Check sheet for the modelled part. Datum: model origin and axes. Units: mm. Face numbers are marked on the shaded views. A direction names the side the tool comes from. Give positions to 0.01 mm unless a question says otherwise; leave off trailing zeros. Write each loop counter-clockwise with the first axis right and the second up, starting at its lowest first coordinate (ties: lowest second). Pieces come first, ordered by that corner, then holes. Notation, with made-up numbers: (-6, 2.25) -> (37, 2.25) arc R17 ccw to (37, 17.25) -> close; hole circle Ø10 at (39.5, 88). An arc over 180 degrees is marked (long way). Return JSON: item names as keys, results as strings.
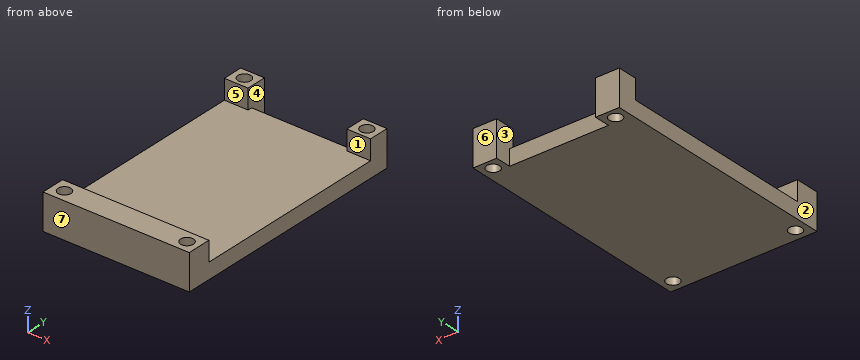
from build123d import *

# Parameters (mm, degrees)
SKETCH1_R           = 3.25
BOSS_EXTRUDE1_DEPTH = 8
SKETCH4_R           = 3.25
BOSS_EXTRUDE3_DEPTH = 10
BOSS_EXTRUDE4_DEPTH = 54
BOSS_EXTRUDE5_DEPTH = 2
BOSS_EXTRUDE6_DEPTH = 2
BOSS_EXTRUDE7_DEPTH = 2
BOSS_EXTRUDE8_DEPTH = 2
SKETCH10_W          = 74
SKETCH10_H          = 18
BOSS_EXTRUDE9_DEPTH = 2


with BuildPart() as part:
    # Sketch1 → Boss-Extrude1 (new body)
    with BuildSketch(Plane.XY):
        Polygon((-27, 52.55), (-27, 60.55), (-35, 60.55), (-35, -60.55), (-27, -60.55), (-27, -52.55), (27, -52.55), (27, -60.55), (35, -60.55), (35, 60.55), (27, 60.55), (27, 52.55), align=None)
        with Locations((31, 55.45)):
            Circle(SKETCH1_R, mode=Mode.SUBTRACT)
        with Locations((-31, 55.45)):
            Circle(SKETCH1_R, mode=Mode.SUBTRACT)
        with Locations((-31, -56.55)):
            Circle(SKETCH1_R, mode=Mode.SUBTRACT)
        with Locations((31, -56.55)):
            Circle(SKETCH1_R, mode=Mode.SUBTRACT)
    extrude(amount=BOSS_EXTRUDE1_DEPTH)

    # Sketch4 → Boss-Extrude3 (add)
    # profile 1 of 4: a face of its own
    with BuildSketch(Plane.XY.offset(8)):
        Polygon((-27, 60.55), (-35, 60.55), (-35, 50.35), (-27, 50.35), (-27, 52.55), align=None)
        with Locations((-31, 55.45)):
            Circle(SKETCH4_R, mode=Mode.SUBTRACT)
    # profile 2 of 4: a face of its own
    with BuildSketch(Plane.XY.offset(8)):
        Polygon((35, 50.35), (35, 60.55), (27, 60.55), (27, 52.55), (27, 50.35), align=None)
        with Locations((31, 55.45)):
            Circle(SKETCH4_R, mode=Mode.SUBTRACT)
    # profile 3 of 4: a face of its own
    with BuildSketch(Plane.XY.offset(8)):
        Polygon((35, -60.55), (35, -50.35), (27, -50.35), (27, -52.55), (27, -60.55), align=None)
        with Locations((31, -56.55)):
            Circle(SKETCH4_R, mode=Mode.SUBTRACT)
    # profile 4 of 4: a face of its own
    with BuildSketch(Plane.XY.offset(8)):
        Polygon((-27, -50.35), (-35, -50.35), (-35, -60.55), (-27, -60.55), (-27, -52.55), align=None)
        with Locations((-31, -56.55)):
            Circle(SKETCH4_R, mode=Mode.SUBTRACT)
    extrude(amount=BOSS_EXTRUDE3_DEPTH)

    # Sketch5 → Boss-Extrude4 (add)
    with BuildSketch(Plane(origin=(-27, 0, 0), x_dir=(0, 0, -1), z_dir=(1, 0, 0))):
        Polygon((-18, -50.35), (-8, -50.35), (-8, -52.55), (0, -52.55), (0, -60.55), (-18, -60.55), align=None)
    extrude(amount=BOSS_EXTRUDE4_DEPTH)

    # Sketch6 → Boss-Extrude5 (add)
    with BuildSketch(Plane(origin=(35, 0, 0), x_dir=(0, 0, -1), z_dir=(1, 0, 0))):
        Polygon((0, -60.55), (0, 60.55), (-18, 60.55), (-18, 50.35), (-8, 50.35), (-8, -50.35), (-18, -50.35), (-18, -60.55), align=None)
    extrude(amount=BOSS_EXTRUDE5_DEPTH)

    # Sketch7 → Boss-Extrude6 (add)
    with BuildSketch(Plane.ZY.offset(-27)):
        Polygon((0, 60.55), (0, 52.55), (8, 52.55), (8, 50.35), (18, 50.35), (18, 60.55), align=None)
    extrude(amount=BOSS_EXTRUDE6_DEPTH)

    # Sketch8 → Boss-Extrude7 (add)
    with BuildSketch(Plane.ZY.offset(35)):
        Polygon((0, 60.55), (0, -60.55), (18, -60.55), (18, -50.35), (8, -50.35), (8, 50.35), (18, 50.35), (18, 60.55), align=None)
    extrude(amount=BOSS_EXTRUDE7_DEPTH)

    # Sketch9 → Boss-Extrude8 (add)
    with BuildSketch(Plane(origin=(-27, 0, 0), x_dir=(0, 0, -1), z_dir=(1, 0, 0))):
        Polygon((0, 52.55), (0, 60.55), (-18, 60.55), (-18, 50.35), (-8, 50.35), (-8, 52.55), align=None)
    extrude(amount=BOSS_EXTRUDE8_DEPTH)

    # Sketch10 → Boss-Extrude9 (add)
    with BuildSketch(Plane.XZ.offset(60.55)):
        with Locations((0, 9)):
            Rectangle(SKETCH10_W, SKETCH10_H)
    extrude(amount=BOSS_EXTRUDE9_DEPTH)


solid = part.part
(1) Set-up check for the marked faces 1, 2 and 3: record each of +Z, -Z, +X, -X, +Y, -Y from which the full face is reachable in a straight line by a thin tool's end or side.
Reply:
{"face 1": "+Z, +X, -X", "face 2": "+Z, -Z, -X, +Y, -Y", "face 3": "+Z, +Y"}
(2) Depth check by flat-ended pin: pin 1 Ø6 at (x, y) = (31, 55.45) entering from -Z; pin 2 Ø8 at (x, z) = (-5, 11.5) entering from +Y; pin 3 Ø4 at (x, y) = (19.5, -15) entering from +Z. Enter the tip coordinate at first touch or a pass-through.
Reply:
{"pin 1": "through", "pin 2": "y = 52.55", "pin 3": "z = 8"}
(3) Cross-section at A-A on x = 31. Enter the section's corners in (y, z), then the cut area to 3 significant figures.
Reply:
{"outline": "(-62.55, 0) -> (-59.8, 0) -> (-59.8, 18) -> (-62.55, 18) -> close; (-53.3, 0) -> (52.2, 0) -> (52.2, 18) -> (50.35, 18) -> (50.35, 8) -> (-50.35, 8) -> (-50.35, 18) -> (-53.3, 18) -> close; (58.7, 0) -> (60.55, 0) -> (60.55, 18) -> (58.7, 18) -> close", "area": "975 mm^2"}
(4) Thickness scan on L1, parallel to Y at x = -31, z = 5.75; L2, parallel to Y at x = -31, z = 8.5; L3, parallel to Y at x = 30, z = 9. Record the ranges inside material, lowest first.
Reply:
{"L1": "-62.55 to -59.8, -53.3 to 52.2, 58.7 to 60.55", "L2": "-62.55 to -59.8, -53.3 to -50.35, 50.35 to 52.2, 58.7 to 60.55", "L3": "-62.55 to -59.64, -53.46 to -50.35, 50.35 to 52.36, 58.54 to 60.55"}
(5) Cross-section at B-B on z = 16.5. Enter the section's corners in (x, y).
Reply:
{"outline": "(-37, -62.55) -> (37, -62.55) -> (37, -50.35) -> (-37, -50.35) -> close; (-37, 50.35) -> (-25, 50.35) -> (-25, 60.55) -> (-37, 60.55) -> close; (25, 50.35) -> (37, 50.35) -> (37, 60.55) -> (25, 60.55) -> close; hole circle Ø6.5 at (-31, -56.55); hole circle Ø6.5 at (-31, 55.45); hole circle Ø6.5 at (31, -56.55); hole circle Ø6.5 at (31, 55.45)"}
(6) Cross-section at D-D on y = -56.55. Enter the section's corners in (x, z), then the cut area to 3 significant figures.
Reply:
{"outline": "(-37, 0) -> (-34.25, 0) -> (-34.25, 18) -> (-37, 18) -> close; (-27.75, 0) -> (27.75, 0) -> (27.75, 18) -> (-27.75, 18) -> close; (34.25, 0) -> (37, 0) -> (37, 18) -> (34.25, 18) -> close", "area": "1,100 mm^2"}
(7) Cross-section at C-C on y = 55.45. Enter the section's corners in (x, z), then the cut area to 3 significant figures.
Reply:
{"outline": "(-37, 0) -> (-34.25, 0) -> (-34.25, 18) -> (-37, 18) -> close; (-27.75, 0) -> (-25, 0) -> (-25, 18) -> (-27.75, 18) -> close; (25, 0) -> (27.75, 0) -> (27.75, 18) -> (25, 18) -> close; (34.25, 0) -> (37, 0) -> (37, 18) -> (34.25, 18) -> close", "area": "198 mm^2"}
(8) Release check for a two-part mould opening along Y. For the marked faces 4, 5, 6 and 7 record: pulls with the +Y half, pulls with the -Y half, needs draft (parallel to the pull), parting line crosses it, or undercut.
Reply:
{"face 4": "needs draft", "face 5": "undercut", "face 6": "pulls with the +Y half", "face 7": "pulls with the -Y half"}
